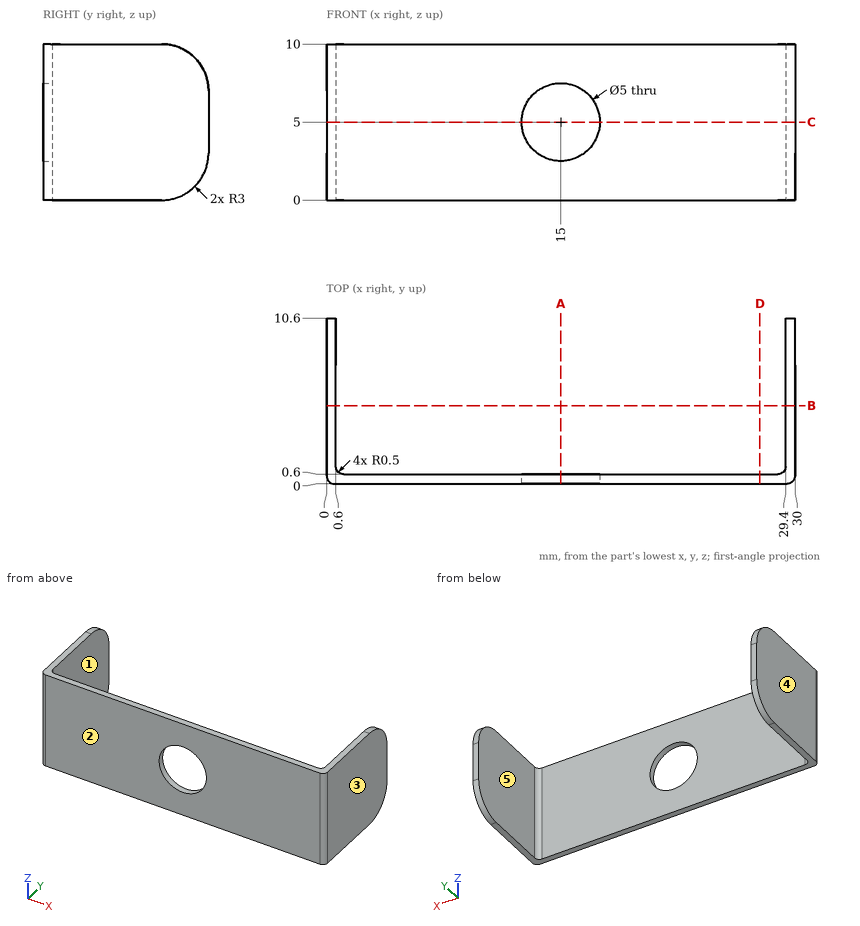
The drawing under review shows one solid part. Ordinate dimensions are in mm from its lowest x, y, z. A direction names the side the tool comes from. Round coordinates to 2 decimals unless told otherwise and drop trailing zeros. Write each loop counter-clockwise with the first axis right and the second up, starting at its lowest first coordinate (ties: lowest second). Pieces come first, ordered by that corner, then holes. Notation, with made-up numbers: M 5.5,-5.5 L 17.5,-5.5 A16 cw 17.5,3.5 Z; hole C 50.25,53.5 d7. An arc over 180 degrees is marked long. One line per item, written item: value. Start each with the question number.
(1) We need section C-C (z = 5). Give the boundary of the cut face in (x, y), and give its area (3 significant figures).
(2) We need section B-B (y = 5). Give the boundary of the cut face in (x, z).
(3) Insertion check: pin 1 (3 mm diameter, centred on x = 13.5, z = 6, fed in from -Y); pin 2 (5 mm diameter, centred on x = 20, z = 5.5, fed in from +Y); pin 3 (1.5 mm diameter, centred on x = 18, y = 2.5, fed in from -Z) (3 decimals). Each pin has a flat end and moves straight along its axis. Give the tip position at first contact, or say it passes through.
(4) Wall thickness on line 1 (X direction, y = 0.55, z = 5); line 2 (X direction, y = 1.5, z = 1.25); line 3 (Z direction, x = 15, y = 0.3): over which ranges is each line inside the solid? List them lowest first.
(5) Machinability: for the marked faces 4 and 5, which of the approach directions +Z, -Z, +X, -X, +Y, -Y give a long, thin tool a straight path to every point of the face, cutting with its end or side? Answer none if there is none.
(6) The part is to be moulded in two halves that separate along X. For the marked faces 1, 2 and 3, say which applies: released by +X, released by -X, zero draft, split by the parting line, or undercut.
(7) We need section A-A (x = 15). Give the boundary of the cut face in (y, z), and give its area (3 significant figures).
(8) We need section D-D (x = 27.75). Give the boundary of the cut face in (y, z).
Result:
1. outline: M 0,0.5 A0.5 ccw 0.5,0 L 12.5,0 L 12.5,0.6 L 1.1,0.6 A0.5 cw 0.6,1.1 L 0.6,10.6 L 0,10.6 Z; M 17.5,0 L 29.5,0 A0.5 ccw 30,0.5 L 30,10.6 L 29.4,10.6 L 29.4,1.1 A0.5 cw 28.9,0.6 L 17.5,0.6 Z
1. area: 27.0 mm²
2. outline: M 0,0 L 0.6,0 L 0.6,10 L 0,10 Z; M 29.4,0 L 30,0 L 30,10 L 29.4,10 Z
3. pin 1: y = 0
3. pin 2: y = 0.6
3. pin 3: through
4. line 1: 0 to 12.5, 17.5 to 30
4. line 2: 0 to 0.6, 29.4 to 30
4. line 3: 0 to 2.5, 7.5 to 10
5. face 4: +Z, -Z, -X, +Y, -Y
5. face 5: +Z, -Z, +Y
6. face 1: undercut
6. face 2: zero draft
6. face 3: released by +X
7. outline: M 0,0 L 0.6,0 L 0.6,2.5 L 0,2.5 Z; M 0,7.5 L 0.6,7.5 L 0.6,10 L 0,10 Z
7. area: 3.00 mm²
8. outline: M 0,0 L 0.6,0 L 0.6,10 L 0,10 Z
